Geometry check sheet. Reference: drawing and pictorial views, mm from the part's lowest x, y, z. A direction names the side the tool comes from. Give positions to 0.01 mm unless a question says otherwise; leave off trailing zeros. Loops run counter-clockwise (first coordinate to the right, second up) from the corner with the lowest first, then second, coordinate; pieces in that order, holes last. Notation, with made-up numbers: (79.5, 75) -> (134.5, 75) arc R20 cw to (134.5, 81) -> close; hole circle Ø5 at (23, -18). An arc over 180 degrees is marked (long way). Answer in a Markdown table with one row per item. Add a question column.
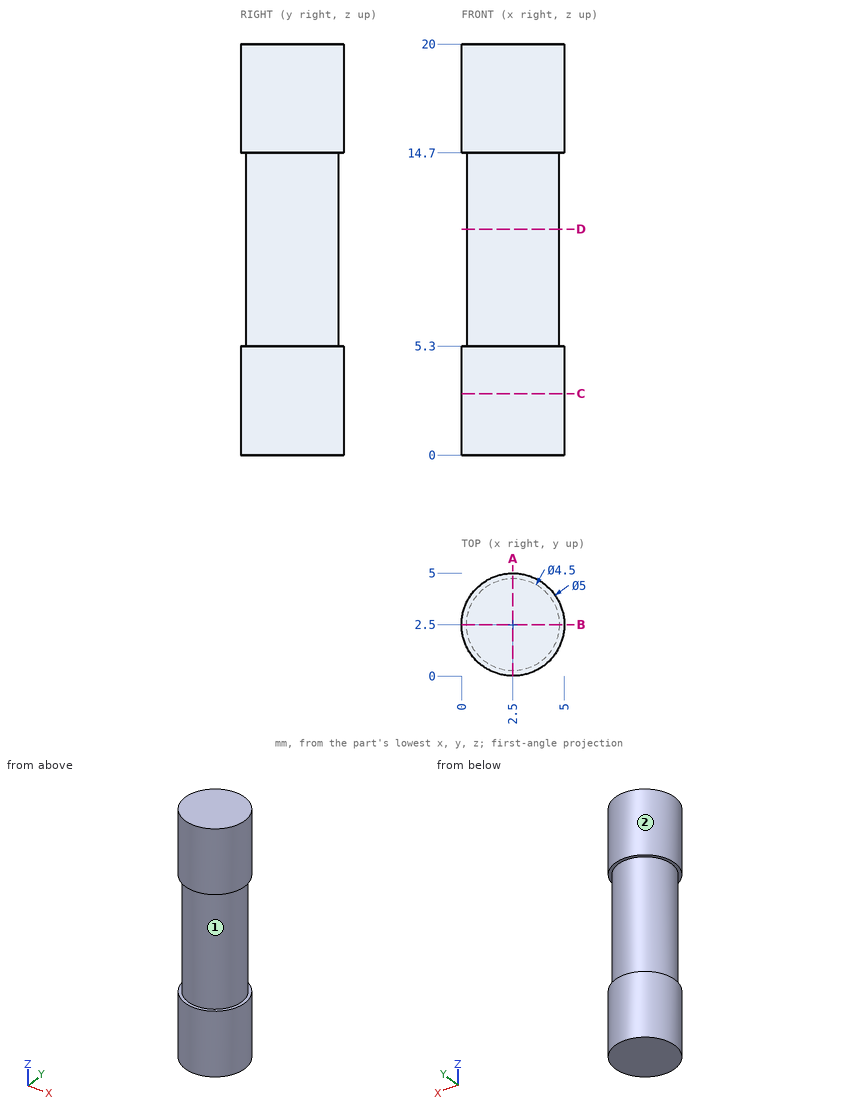
1. Sectioned sample at D-D (z = 11). Enter the section's corners in (x, y).
2. Sectioned sample at C-C (z = 3). Enter the section's corners in (x, y), plus the area to 3 significant figures.
3. Access from +Z, -Z, +X, -X, +Y, -Y to the whole of each face (thin tool, end or side, straight path). Record for the marked faces 1 and 2.
4. Sectioned sample at A-A (x = 2.5). Enter the section's corners in (y, z).
5. Gauge pin test, flat end, axial feed: pin 1 Ø3 at (y, z) = (1.5, 5) entering from +X. Record the tip position at first contact, or that the pin passes through.
6. Material ranges on L1, parallel to Z at x = 4.25, y = 0.8; L2, parallel to X at y = 2.55, z = 6.25; L3, parallel to Y at x = 2.6, z = 17.25, recorded low to high. Write a range as from..to.
Response:
| question | item | result |
|---|---|---|
| 1 | outline | circle Ø4.5 at (2.5, 2.5) |
| 2 | outline | circle Ø5 at (2.5, 2.5) |
| 2 | area | 19.6 mm2 |
| 3 | face 1 | none |
| 3 | face 2 | +Z, -Z |
| 4 | outline | (0, 0) -> (5, 0) -> (5, 5.3) -> (4.75, 5.3) -> (4.75, 14.7) -> (5, 14.7) -> (5, 20) -> (0, 20) -> (0, 14.7) -> (0.25, 14.7) -> (0.25, 5.3) -> (0, 5.3) -> close |
| 5 | pin 1 | stops at x = 5 |
| 6 | L1 | z = 0..5.3, 14.7..20 |
| 6 | L2 | x = 0.25..4.75 |
| 6 | L3 | y = 0..5 |
